Here's the drawing with two shaded views (mm, measured from the low corner). I have some questions. Coordinates: 2 decimals unless noted, no trailing zeros. Order: outer loops, then holes, each group sorted by start corner. A loop starts at its lowest first (then second) coordinate and runs counter-clockwise, first axis right, second up. Notation, with made-up numbers: (58, 12) -> (75, 12) arc R18 ccw to (75, 44) -> close; hole circle Ø6 at (-28, -24). An arc over 180 degrees is marked (long way). Answer in a Markdown table with one row per item. Add a question column.
1. Will these pins go through, and if not, where does the flat tip stop? pin 1 (3 mm diameter, centred on y = 3, z = 5, fed in from -X); pin 2 (1.6 mm diameter, centred on y = 3, z = 78, fed in from +X).
2. If I drill on line 1 along X through (y, z) = (4.55, 72); line 2 along Z through (x, y) = (78, 3.5), over which ranges is the centre line in solid material (lowest first)? Write a range as [from, to].
3. Imagine slicing it at A-A on x = 6. Write out the boundary of the cut face in (y, z).
4. Imagine slicing it at B-B on z = 12. Write out the boundary of the cut face in (x, y).
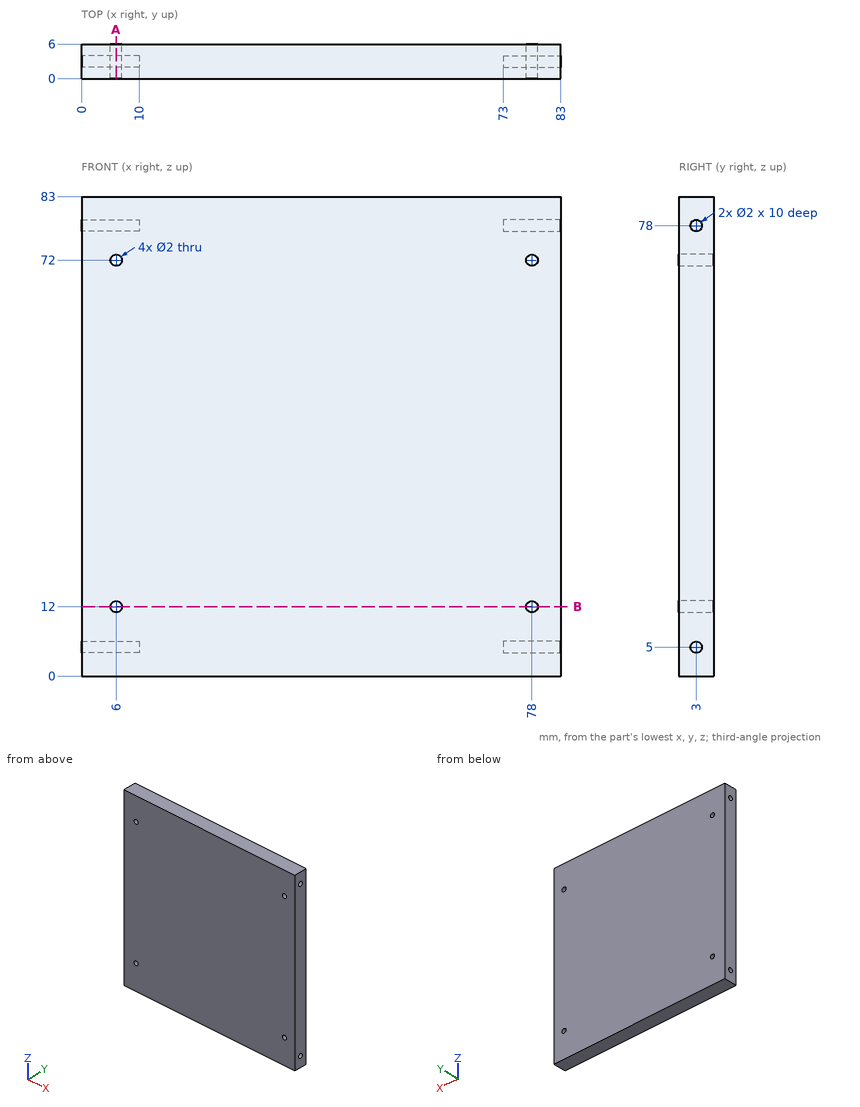
Answers follow:
| question | item | result |
|---|---|---|
| 1 | pin 1 | stops at x = 0 |
| 1 | pin 2 | stops at x = 73 |
| 2 | line 1 | x = [0, 5], [7, 77], [79, 83] |
| 2 | line 2 | z = [0, 4.13], [5.87, 11], [13, 71], [73, 77.13], [78.87, 83] |
| 3 | outline | (0, 0) -> (6, 0) -> (6, 11) -> (0, 11) -> close; (0, 13) -> (6, 13) -> (6, 71) -> (0, 71) -> close; (0, 73) -> (6, 73) -> (6, 83) -> (0, 83) -> close; hole circle Ø2 at (3, 5); hole circle Ø2 at (3, 78) |
| 4 | outline | (0, 0) -> (5, 0) -> (5, 6) -> (0, 6) -> close; (7, 0) -> (77, 0) -> (77, 6) -> (7, 6) -> close; (79, 0) -> (83, 0) -> (83, 6) -> (79, 6) -> close |
